```python
from build123d import *

# Parameters (mm, degrees)
SKETCH1_W                   = 24
SKETCH1_H                   = 75
BOSS_EXTRUDE1_DEPTH         = 3
SKETCH2_W                   = 11
SKETCH2_H                   = 75
BOSS_EXTRUDE2_DEPTH         = 7.5
TAP_DRILL_FOR_M3X0_5_TAP1_D = 2.5
SKETCH5_W                   = 7
SKETCH5_H                   = 72.5
CUT_EXTRUDE1_DEPTH          = 6
CUT_LOFT1_START             = 11.622950039
CUT_LOFT1_DEPTH             = 8.5
CUT_LOFT5_START             = 27.122950039
CUT_LOFT5_DEPTH             = 8.5
SKETCH16_W                  = 24
SKETCH16_H                  = 2.5
BOSS_EXTRUDE4_DEPTH         = 13.5
SKETCH17_W                  = 5
SKETCH17_H                  = 7.5
BOSS_EXTRUDE5_DEPTH         = 7
SKETCH18_R                  = 2
CUT_EXTRUDE2_DEPTH          = 7.5
SKETCH20_W                  = 5
SKETCH20_H                  = 5
CUT_EXTRUDE3_DEPTH          = 2


# Read off the part's stored shape, not the designer's step: Cut-Loft1, Cut-Loft5
with BuildPart() as part:
    # Sketch1 → Boss-Extrude1 (new body)
    with BuildSketch(Plane.XY):
        with Locations((23.622950039, -13.56022481)):
            Rectangle(SKETCH1_W, SKETCH1_H)
    extrude(amount=BOSS_EXTRUDE1_DEPTH)

    # Sketch2 → Boss-Extrude2 (add)
    with BuildSketch(Plane.XY.offset(3)):
        with Locations((23.622950039, -13.56022481)):
            Rectangle(SKETCH2_W, SKETCH2_H)
    extrude(amount=BOSS_EXTRUDE2_DEPTH)

    # Tap Drill for M3x0.5 Tap1 (through all)
    with Locations(Plane(origin=(23.622950039, 16.43977519, 10.5), x_dir=(1, 0, 0), z_dir=(0, 0, 1))):
        with Locations((0, 0), (0, -15), (0, -30), (0, -45), (0, -60)):
            Hole(TAP_DRILL_FOR_M3X0_5_TAP1_D / 2)

    # Sketch5 → Cut-Extrude1 (cut)
    with BuildSketch(Plane(origin=(0, 0, 0), x_dir=(-1, 0, 0), z_dir=(0, 0, -1))):
        with Locations((-23.622950039, -14.81022481)):
            Rectangle(SKETCH5_W, SKETCH5_H)
    extrude(amount=-CUT_EXTRUDE1_DEPTH, mode=Mode.SUBTRACT)

    # Cut-Loft1 outline → Cut-Loft1 (cut)
    with BuildSketch(Plane.YZ.offset(CUT_LOFT1_START)):
        with BuildLine():
            ThreePointArc((-51.06022481, 0.4), (-49.96022481, 1.5), (-51.06022481, 2.6))
            Line((-51.06022481, 2.6), (-51.06022481, 0.4))
        make_face()
    extrude(amount=CUT_LOFT1_DEPTH, mode=Mode.SUBTRACT)

    # Cut-Loft5 outline → Cut-Loft5 (cut)
    with BuildSketch(Plane.YZ.offset(CUT_LOFT5_START)):
        with BuildLine():
            Line((-51.06022481, 2.6), (-51.06022481, 0.4))
            ThreePointArc((-51.06022481, 0.4), (-49.96022481, 1.5), (-51.06022481, 2.6))
        make_face()
    extrude(amount=CUT_LOFT5_DEPTH, mode=Mode.SUBTRACT)

    # Sketch16 → Boss-Extrude4 (add)
    with BuildSketch(Plane(origin=(0, 0, 0), x_dir=(-1, 0, 0), z_dir=(0, 0, -1))):
        with Locations((-23.622950039, 22.68977519)):
            Rectangle(SKETCH16_W, SKETCH16_H)
    extrude(amount=BOSS_EXTRUDE4_DEPTH)

    # Sketch17 → Boss-Extrude5 (add)
    with BuildSketch(Plane(origin=(0, 23.93977519, 0), x_dir=(1, 0, 0), z_dir=(0, 1, 0))):
        with Locations((23.622950039, -6.75)):
            Rectangle(SKETCH17_W, SKETCH17_H)
    extrude(amount=BOSS_EXTRUDE5_DEPTH)

    # Sketch18 → Cut-Extrude2 (cut)
    with BuildSketch(Plane.XY.offset(10.5)):
        with Locations((23.622950039, 27.93977519)):
            Circle(SKETCH18_R)
    extrude(amount=-CUT_EXTRUDE2_DEPTH, mode=Mode.SUBTRACT)

    # Sketch20 → Cut-Extrude3 (cut)
    with BuildSketch(Plane(origin=(0, 23.93977519, 0), x_dir=(1, 0, 0), z_dir=(0, 1, 0))):
        with Locations((23.622950039, 4)):
            Rectangle(SKETCH20_W, SKETCH20_H)
    extrude(amount=-CUT_EXTRUDE3_DEPTH, mode=Mode.SUBTRACT)


solid = part.part
```
Read the model definition and answer for the solid it produces. Units are mm, in the model's axes. A direction names the side the tool comes from. Round coordinates to 2 decimals unless told otherwise and drop trailing zeros. Write each loop counter-clockwise with the first axis right and the second up, starting at its lowest first coordinate (ties: lowest second). Pieces come first, ordered by that corner, then holes. Notation, with made-up numbers: (50.25, 5) -> (92.25, 5) arc R6 cw to (92.25, 11) -> close; hole circle Ø5 at (87, 23). An arc over 180 degrees is marked (long way). Answer in a Markdown table with one row per item. Add a question column.
1) Which of the six approach directions +Z, -Z, +X, -X, +Y, -Y give full straight-line access (tool end or side, diameter ignored) to faces 1 (the face through (25, -14, 6)), 2 (the face through (26.123, 27, 7)), 3 (the face through (16, -14, 0)), 4 (the face through (29.123, -14, 7)), 5 (the face through (18.123, -14, 7))?
2) Find section C-C, the plane y = 20. Determine the outline of the cut face in (x, z), and give its area (4 significant figures).
3) Find section B-B, the plane x = 31.25. Determine the outline of the cut face in (y, z), and give its area (3 significant figures).
4) Determine the mould class of faces 6 (the face through (24, 23, -13.5)), 7 (the face through (31.31, -49.96, 1.48)), 8 (the face through (24, 23.94, -7)) for opening direction Z: pulls with the +Z half, pulls with the -Z half, needs draft (parallel to the pull), parting line crosses it, or undercut.
5) Given P1, Ø1.5, axis at x = 18, z = 0.5, coming from the -Y side; P2, Ø2, axis at y = 26, z = 8, coming from the +X side; P3, Ø5.5, axis at y = 29, z = 5, coming from the -X side; P4, Ø4, axis at y = -6, z = 7, coming from the -X side, each flat-ended and moving along its own axis, determine where each tip first touches the part or whether it passes through.
6) Find section A-A, the plane z = 1.5. Determine the outline of the cut face in (x, y).
7) Consider line 1 (Y direction, x = 13.5, z = -1); line 2 (X direction, y = 9.5, z = 9.5); line 3 (Z direction, x = 26.5, y = -33). Determine where each line is inside the solid, lowest interval first.
Findings below:
| question | item | result |
|---|---|---|
| 1 | face 1 | -Z, -Y |
| 1 | face 2 | +Z, -Z, +X, +Y |
| 1 | face 3 | -Z, +X, -X, -Y |
| 1 | face 4 | +Z, +X, +Y, -Y |
| 1 | face 5 | +Z, -X, +Y, -Y |
| 2 | outline | (11.62, 0) -> (20.12, 0) -> (20.12, 6) -> (27.12, 6) -> (27.12, 0) -> (35.62, 0) -> (35.62, 3) -> (29.12, 3) -> (29.12, 10.5) -> (18.12, 10.5) -> (18.12, 3) -> (11.62, 3) -> close |
| 2 | area | 112.5 mm² |
| 3 | outline | (-51.06, 0) -> (21.44, 0) -> (21.44, -13.5) -> (23.94, -13.5) -> (23.94, 3) -> (-51.06, 3) -> (-51.06, 2.6) arc R1.1 cw to (-51.06, 0.4) -> close |
| 3 | area | 257 mm² |
| 4 | face 6 | pulls with the -Z half |
| 4 | face 7 | undercut |
| 4 | face 8 | needs draft |
| 5 | P1 | y = -51.06 |
| 5 | P2 | x = 26.12 |
| 5 | P3 | x = 21.12 |
| 5 | P4 | x = 18.12 |
| 6 | outline | (11.62, -49.96) -> (20.12, -49.96) -> (20.12, 21.44) -> (27.12, 21.44) -> (27.12, -49.96) -> (35.62, -49.96) -> (35.62, 23.94) -> (11.62, 23.94) -> close |
| 7 | line 1 | 21.44 to 23.94 |
| 7 | line 2 | 18.12 to 29.12 |
| 7 | line 3 | 6 to 10.5 |
